```python
from build123d import *

# Parameters (mm, degrees)
SKETCH1_R           = 8
BOSS_EXTRUDE1_DEPTH = 18
CUT_EXTRUDE1_DEPTH  = 8
SKETCH3_W           = 6.2
SKETCH3_H           = 7.1
CUT_EXTRUDE2_DEPTH  = 8
SKETCH4_W           = 6
SKETCH4_H           = 2.5
CUT_EXTRUDE3_DEPTH  = 20
SKETCH5_R           = 1.2
CUT_EXTRUDE4_DEPTH  = 9


with BuildPart() as part:
    # Sketch1 → Boss-Extrude1 (new body)
    with BuildSketch(Plane(origin=(0, 0, 0), x_dir=(1, 0, 0), z_dir=(0, 1, 0))):
        Circle(SKETCH1_R)
    extrude(amount=BOSS_EXTRUDE1_DEPTH)

    # Sketch2 → Cut-Extrude1 (cut)
    with BuildSketch(Plane.XZ):
        with BuildLine():
            Line((-1.501271778, 1.395952381), (1.501271778, 1.395952381))
            ThreePointArc((1.501271778, 1.395952381), (0, -2.05), (-1.501271778, 1.395952381))
        make_face()
    extrude(amount=-CUT_EXTRUDE1_DEPTH, mode=Mode.SUBTRACT)

    # Sketch3 → Cut-Extrude2 (cut)
    with BuildSketch(Plane(origin=(0, 18, 0), x_dir=(1, 0, 0), z_dir=(0, 1, 0))):
        Rectangle(SKETCH3_W, SKETCH3_H)
    extrude(amount=-CUT_EXTRUDE2_DEPTH, mode=Mode.SUBTRACT)

    # Sketch4 → Cut-Extrude3 (cut)
    with BuildSketch(Plane(origin=(0, 18, 0), x_dir=(1, 0, 0), z_dir=(0, 1, 0))):
        with Locations((0, -5.561582467)):
            Rectangle(SKETCH4_W, SKETCH4_H)
    extrude(amount=-CUT_EXTRUDE3_DEPTH, mode=Mode.SUBTRACT)

    # Sketch5 → Cut-Extrude4 (cut)
    with BuildSketch(Plane.XY.offset(8)):
        with Locations((0, 3.328333926)):
            Circle(SKETCH5_R)
        with Locations((0, 14.225763094)):
            Circle(SKETCH5_R)
    extrude(amount=-CUT_EXTRUDE4_DEPTH, mode=Mode.SUBTRACT)


solid = part.part
```
Source: CAD feature listing. Evaluate the final solid. Frame: model axes, mm. A direction names the side the tool comes from. Round coordinates to 2 decimals unless told otherwise and drop trailing zeros. Loops run counter-clockwise (first coordinate to the right, second up) from the corner with the lowest first, then second, coordinate; pieces in that order, holes last. Notation, with made-up numbers: M 20.25,16.25 L 25.25,16.25 A19 ccw 25.25,33.25 Z; hole C -13,21 d2. An arc over 180 degrees is marked long. Use a Markdown table: item, result. Add a question column.
1. Mould query, pull axis Z, two halves, no side actions, for faces 5 (the cylindrical face through (-1.73, 8.87, 7.81)), 6 (the flat face through (0, 8, 0)), 7 (the cylindrical face through (0.645, 15.238, 3.936)). Classes: pulls with the +Z half, pulls with the -Z half, needs draft (parallel to the pull), parting line crosses it, or undercut.
2. Line query: line 1 (Y direction, x = 0, z = 3.9); line 2 (X direction, y = 3.5, z = 0); line 3 (Z direction, x = -2.75, y = 15.5). Output: solid intervals per line, ascending.
3. Reachability of faces 1 (the cylindrical face through (-1.2, 14.28, 7.41)), 2 (the cylindrical face through (0.07, 3.94, -2.05)), 3 (the flat face through (0, 10, 0)), 4 (the flat face through (3, 9, 6)) from +Z, -Z, +X, -X, +Y, -Y: full face, straight path, thin tool, end or side. Return the list, or none.
4. Section query D-D on y = 9.5. Return the cut outline in (x, z).
5. Section query C-C on z = 1.75. Return the cut outline in (x, y), then the cut area to 3 significant figures.
6. Section query A-A on x = 0. Give the number of separate pieces and of enclosed holes in the cut face, then the cut area to 3 significant figures.
7. Contact query for flat-ended pins moving along their axis: P1, Ø3.5, axis at x = 0.5, y = 3.5, coming from the -Z side; P2, Ø1.5, axis at y = 5.5, z = -3, coming from the -X side; P3, Ø1.7, axis at x = 0, z = 0, coming from the -Y side; P4, Ø2, axis at x = 6, y = 7.5, coming from the +Z side (3 decimals). Output: stop coordinate, or through.
8. Section query B-B on y = 5.5. Return the cut outline in (x, z), then the cut area to 3 significant figures.
Reported:
| question | item | result |
|---|---|---|
| 1 | face 5 | parting line crosses it |
| 1 | face 6 | undercut |
| 1 | face 7 | needs draft |
| 2 | line 1 | y = 0 to 2.13, 4.53 to 13.03, 15.43 to 18 |
| 2 | line 2 | x = -8 to -2.05, 2.05 to 8 |
| 2 | line 3 | z = -7.51 to -3.55, 3.55 to 4.31, 6.81 to 7.51 |
| 3 | face 1 | +Z |
| 3 | face 2 | -Y |
| 3 | face 3 | +Y |
| 3 | face 4 | +Y, -Y |
| 4 | outline | C 0,0 d16; hole M -3,4.31 L 3,4.31 L 3,6.81 L -3,6.81 Z |
| 5 | outline | M -7.81,0 L 7.81,0 L 7.81,18 L 3.1,18 L 3.1,10 L -3.1,10 L -3.1,18 L -7.81,18 Z; hole C 0,3.33 d2.4 |
| 5 | area | 227 mm² |
| 6 | separate pieces | 6 |
| 6 | enclosed holes | 0 |
| 6 | area | 144 mm² |
| 7 | P1 | stops at z = -8 |
| 7 | P2 | stops at x = -7.68 |
| 7 | P3 | stops at y = 8 |
| 7 | P4 | stops at z = 6.245 |
| 8 | outline | C 0,0 d16; hole M -3,4.31 L 3,4.31 L 3,6.81 L -3,6.81 Z; hole M -1.5,1.4 A2.05 ccw long 1.5,1.4 Z |
| 8 | area | 174 mm² |
